from build123d import *

# Parameters (mm, degrees)
SKETCH1_W           = 48
SKETCH1_H           = 100
BOSS_EXTRUDE1_DEPTH = 5
SKETCH2_W           = 20
SKETCH2_H           = 5
BOSS_EXTRUDE2_DEPTH = 5
SKETCH3_R           = 6
BOSS_EXTRUDE3_DEPTH = 5
SKETCH4_R           = 2.5
CUT_EXTRUDE1_DEPTH  = 5


with BuildPart() as part:
    # Sketch1 → Boss-Extrude1 (new body)
    with BuildSketch(Plane.XY):
        Rectangle(SKETCH1_W, SKETCH1_H)
    extrude(amount=BOSS_EXTRUDE1_DEPTH)

    # Sketch2 → Boss-Extrude2 (add)
    with BuildSketch(Plane(origin=(0, 50, 0), x_dir=(1, 0, 0), z_dir=(0, 1, 0))):
        with Locations((0, -2.5)):
            Rectangle(SKETCH2_W, SKETCH2_H)
    boss_extrude2 = extrude(amount=BOSS_EXTRUDE2_DEPTH)

    # Mirror1: Boss-Extrude2 across plane
    add(boss_extrude2.mirror(Plane.ZX))

    # Sketch3 → Boss-Extrude3 (add)
    with BuildSketch(Plane.XY.offset(5)):
        with Locations((0, 52.5)):
            Circle(SKETCH3_R)
    boss_extrude3 = extrude(amount=-BOSS_EXTRUDE3_DEPTH)

    # Sketch4 → Cut-Extrude1 (cut)
    with BuildSketch(Plane.XY.offset(5)):
        with Locations((0, 52.5)):
            Circle(SKETCH4_R)
    cut_extrude1 = extrude(amount=-CUT_EXTRUDE1_DEPTH, mode=Mode.SUBTRACT)

    # Mirror2: Boss-Extrude3, Cut-Extrude1 across plane
    add(boss_extrude3.mirror(Plane.ZX))
    add(cut_extrude1.mirror(Plane.ZX), mode=Mode.SUBTRACT)


solid = part.part
Work out the finished part from the listing and answer in its coordinate system (mm). A direction names the side the tool comes from. Round coordinates to 2 decimals unless told otherwise and drop trailing zeros. Write each loop counter-clockwise with the first axis right and the second up, starting at its lowest first coordinate (ties: lowest second). Pieces come first, ordered by that corner, then holes. Notation, with made-up numbers: (7, 48) -> (65, 48) arc R5 cw to (65, 55) -> close; hole circle Ø9 at (83.25, -33). An arc over 180 degrees is marked (long way). Write each question's results on one line, items separated by ' | '.
Item 1: A cutting plane is placed at A-A, the plane x = 0. Determine the outline of the cut face in (y, z).
Result set:
outline: (-58.5, 0) -> (-55, 0) -> (-55, 5) -> (-58.5, 5) -> close; (-50, 0) -> (50, 0) -> (50, 5) -> (-50, 5) -> close; (55, 0) -> (58.5, 0) -> (58.5, 5) -> (55, 5) -> close
Item 2: A cutting plane is placed at C-C, the plane z = 3.55. Determine the outline of the cut face in (x, y), plus the area to 3 significant figures.
Result set:
outline: (-24, -50) -> (-10, -50) -> (-10, -55) -> (-5.45, -55) arc R6 ccw to (5.45, -55) -> (10, -55) -> (10, -50) -> (24, -50) -> (24, 50) -> (10, 50) -> (10, 55) -> (5.45, 55) arc R6 ccw to (-5.45, 55) -> (-10, 55) -> (-10, 50) -> (-24, 50) -> close; hole circle Ø5 at (0, -52.5); hole circle Ø5 at (0, 52.5) | area: 5,020 mm^2
Item 3: Find the intervals of material crossed by line 1 along Y through (x, z) = (0, 1.9); line 2 along X through (y, z) = (-52.5, 3.2); line 3 along Y through (x, z) = (9.5, 4.65), in increasing order. Write a range as [from, to].
Result set:
line 1: [-58.5, -55], [-50, 50], [55, 58.5] | line 2: [-10, -2.5], [2.5, 10] | line 3: [-55, 55]
Item 4: Which of the six approach directions +Z, -Z, +X, -X, +Y, -Y give full straight-line access (tool end or side, diameter ignored) to faces 1 (the face through (10, -52, 3)), 2 (the face through (-10, -52, 3)), 3 (the face through (10, 52, 3)), 4 (the face through (-10, 52, 3))?
Result set:
face 1: +Z, -Z, +X, -Y | face 2: +Z, -Z, -X, -Y | face 3: +Z, -Z, +X, +Y | face 4: +Z, -Z, -X, +Y
Item 5: Flat-ended cylindrical pins translate along their axes: P1, Ø2, axis at x = 2.5, y = -13, coming from the -Z side; P2, Ø2.5, axis at y = -52, z = 2, coming from the +X side; P3, Ø1.5, axis at x = -15, z = 3.5, coming from the -Y side; P4, Ø3, axis at x = 0, y = 52.5, coming from the -Z side. Find the tip coordinate at first contact, or state that the pin passes through.
Result set:
P1: z = 0 | P2: x = 10 | P3: y = -50 | P4: through
Item 6: A cutting plane is placed at D-D, the plane x = 14. Determine the outline of the cut face in (y, z).
Result set:
outline: (-50, 0) -> (50, 0) -> (50, 5) -> (-50, 5) -> close
Item 7: A cutting plane is placed at B-B, the plane y = -52.5. Determine the outline of the cut face in (x, z), plus the area to 3 significant figures.
Result set:
outline: (-10, 0) -> (-2.5, 0) -> (-2.5, 5) -> (-10, 5) -> close; (2.5, 0) -> (10, 0) -> (10, 5) -> (2.5, 5) -> close | area: 75.0 mm^2
